For this review, take the finished solid that the model builds, in its own axes (mm). Face numbers are marked on the shaded views. A direction names the side the tool comes from. Coordinates: 2 decimals unless noted, no trailing zeros. Loops run counter-clockwise (first coordinate to the right, second up) from the corner with the lowest first, then second, coordinate; pieces in that order, holes last. Notation, with made-up numbers: (88, 12.5) -> (138, 12.5) arc R30 cw to (138, 45.5) -> close; hole circle Ø10 at (58, 16). An arc over 180 degrees is marked (long way). Answer in a Markdown table with one row per item.
from build123d import *

# Parameters (mm, degrees)
SKETCH3_R           = 2.25
BOSS_EXTRUDE1_DEPTH = 12
INNER_EDGES_R       = 0.5
CUT_EXTRUDE2_DEPTH  = 13
OUTER_EDGES_R       = 0.5


with BuildPart() as part:
    # Sketch3 → Boss-Extrude1 (new body)
    with BuildSketch(Plane.XY):
        Polygon((-2.5, 15), (2.5, 15), (2.5, 6.035533906), (8.838834765, 12.374368671), (12.374368671, 8.838834765), (6.035533906, 2.5), (15, 2.5), (15, -2.5), (6.035533906, -2.5), (12.374368671, -8.838834765), (8.838834765, -12.374368671), (2.5, -6.035533906), (2.5, -15), (-2.5, -15), (-2.5, -6.035533906), (-8.838834765, -12.374368671), (-12.374368671, -8.838834765), (-6.035533906, -2.5), (-15, -2.5), (-15, 2.5), (-6.035533906, 2.5), (-12.374368671, 8.838834765), (-8.838834765, 12.374368671), (-2.5, 6.035533906), align=None)
        Circle(SKETCH3_R, mode=Mode.SUBTRACT)
    extrude(amount=BOSS_EXTRUDE1_DEPTH)

    # Inner Edges
    inner_edges_edges = [part.edges().sort_by_distance(p)[0] for p in [
        (6.035533906, 2.5, 6),
        (6.035533906, -2.5, 6),
        (2.5, -6.035533906, 6),
        (-2.5, -6.035533906, 6),
        (-6.035533906, -2.5, 6),
        (-6.035533906, 2.5, 6),
        (-2.5, 6.035533906, 6),
        (2.5, 6.035533906, 6),
    ]]
    fillet(inner_edges_edges, radius=INNER_EDGES_R)

    # Sketch4 → Cut-Extrude2 (cut, through all)
    with BuildSketch(Plane.XY.offset(12)):
        Polygon((10.960155108, -7.424621202), (10.606601718, -10.606601718), (12.374368671, -8.838834765), align=None)
        Polygon((13, 2.5), (15, 0), (15, 2.5), align=None)
        Polygon((8.838834765, 12.374368671), (7.424621202, 10.960155108), (10.606601718, 10.606601718), align=None)
        Polygon((-2.5, 13), (0, 15), (-2.5, 15), align=None)
        Polygon((-10.960155108, 7.424621202), (-10.606601718, 10.606601718), (-12.374368671, 8.838834765), align=None)
        Polygon((-13, -2.5), (-15, 0), (-15, -2.5), align=None)
        Polygon((-7.424621202, -10.960155108), (-10.606601718, -10.606601718), (-8.838834765, -12.374368671), align=None)
        Polygon((0, -15), (2.5, -15), (2.5, -13), align=None)
    extrude(amount=-CUT_EXTRUDE2_DEPTH, mode=Mode.SUBTRACT)

    # Outer Edges
    outer_edges_edges = [part.edges().sort_by_distance(p)[0] for p in [
        (13, 2.5, 6),
        (15, 0, 6),
        (10.606601718, 10.606601718, 6),
        (7.424621202, 10.960155108, 6),
        (-2.5, 13, 6),
        (0, 15, 6),
        (-10.960155108, 7.424621202, 6),
        (-10.606601718, 10.606601718, 6),
        (-13, -2.5, 6),
        (-15, 0, 6),
        (-10.606601718, -10.606601718, 6),
        (-7.424621202, -10.960155108, 6),
        (2.5, -13, 6),
        (0, -15, 6),
        (10.960155108, -7.424621202, 6),
        (10.606601718, -10.606601718, 6),
        (12.374368671, 8.838834765, 6),
        (15, -2.5, 6),
        (8.838834765, -12.374368671, 6),
        (-2.5, -15, 6),
        (-12.374368671, -8.838834765, 6),
        (-15, 2.5, 6),
        (-8.838834765, 12.374368671, 6),
        (2.5, 15, 6),
    ]]
    fillet(outer_edges_edges, radius=OUTER_EDGES_R)


solid = part.part
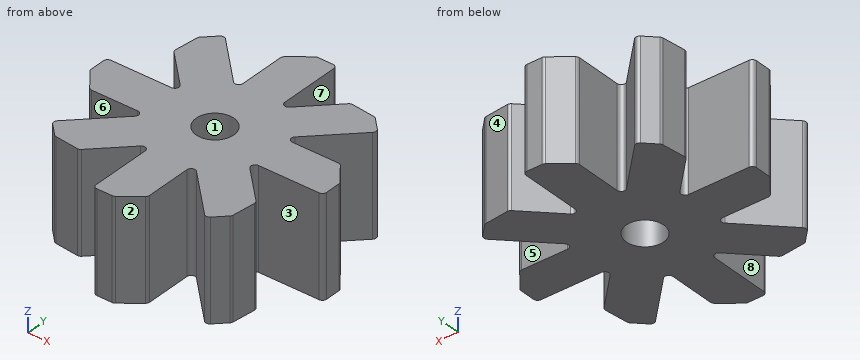
Item 1: For L1, parallel to Y at x = 10.25, z = 3.5; L2, parallel to X at y = 7.25, z = 2.5; L3, parallel to Y at x = 0, z = 6, list the stretches that pass through material, from the lowest coordinate up.
Worked answers:
| item | result |
|---|---|
| L1 | -10.96 to -6.71, -2.5 to 2.5, 6.71 to 10.65 |
| L2 | -10.79 to -3.71, -2.5 to 2.5, 3.71 to 10.79 |
| L3 | -14.97 to -2.25, 2.25 to 14.97 |
Item 2: The part is to be moulded in two halves that separate along X. For the marked faces 1, 2 and 3, say which applies: +X half, -X half, draft (parallel to the pull), parting line (faces both ways), or undercut.
Worked answers:
| item | result |
|---|---|
| face 1 | undercut |
| face 2 | +X half |
| face 3 | draft |
Item 3: Take a section at A-A, the plane x = -9.75. State the section outline as (y, z) points, and give its area (3 significant figures).
Worked answers:
| item | result |
|---|---|
| outline | (-10.7, 0) -> (-6.21, 0) -> (-6.21, 12) -> (-10.7, 12) -> close; (-2.5, 0) -> (2.5, 0) -> (2.5, 12) -> (-2.5, 12) -> close; (6.21, 0) -> (11.46, 0) -> (11.46, 12) -> (6.21, 12) -> close |
| area | 177 mm² |
Item 4: Insertion check: pin 1 (1.7 mm diameter, centred on x = -9.5, z = 8, fed in from -Y); pin 2 (6 mm diameter, centred on x = 9, z = 6.5, fed in from +Y); pin 3 (6 mm diameter, centred on y = 11.5, z = 7.5, fed in from +X). Each pin has a flat end and moves straight along its axis. Give the tip position at first contact, or say it passes through.
Worked answers:
| item | result |
|---|---|
| pin 1 | y = -10.82 |
| pin 2 | y = 10.94 |
| pin 3 | x = 12.17 |
Item 5: Take a section at B-B, the plane x = -3. State the section outline as (y, z) points.
Worked answers:
| item | result |
|---|---|
| outline | (-6.74, 0) -> (6.74, 0) -> (6.74, 12) -> (-6.74, 12) -> close |
Item 6: Take a section at C-C, the plane y = -5. State the section outline as (x, z) points, and give its area (3 significant figures).
Worked answers:
| item | result |
|---|---|
| outline | (-8.54, 0) -> (8.54, 0) -> (8.54, 12) -> (-8.54, 12) -> close |
| area | 205 mm² |
Item 7: For the marked faces 4, 5, 6, 7 and 8, list the 3-axis set-ups (+Z, -Z, +X, -X, +Y, -Y) from which the entire face can be reached by the end or side of a thin tool; tool diameter is ignored.
Worked answers:
| item | result |
|---|---|
| face 4 | +Z, -Z, +X, +Y |
| face 5 | +Z, -Z, +X |
| face 6 | +Z, -Z, -X |
| face 7 | +Z, -Z, +Y |
| face 8 | +Z, -Z, -Y |
